Part model, mm, in its own coordinate system. A direction names the side the tool comes from. Coordinates: 2 decimals unless noted, no trailing zeros. Write each loop counter-clockwise with the first axis right and the second up, starting at its lowest first coordinate (ties: lowest second). Pieces come first, ordered by that corner, then holes. Notation, with made-up numbers: (35, 75) -> (66, 75) arc R26 cw to (66, 110) -> close; hole circle Ø10 at (-6.5, 19.5). An arc over 180 degrees is marked (long way). Write item = value, one per line.
from build123d import *

# Parameters (mm, degrees)
IZIM1_W                     = 40
IZIM1_H                     = 70
Y_KSEKLIK_EKSTR_ZYON1_DEPTH = 20
IZIM2_W                     = 18
IZIM2_H                     = 10
KES_EKSTR_ZYON1_DEPTH       = 71
IZIM3_W                     = 40
IZIM3_H                     = 20
Y_KSEKLIK_EKSTR_ZYON2_DEPTH = 5
IZIM4_W                     = 40
IZIM4_H                     = 20
Y_KSEKLIK_EKSTR_ZYON3_DEPTH = 20
IZIM5_W                     = 16
IZIM5_H                     = 10
KES_EKSTR_ZYON2_DEPTH       = 21


with BuildPart() as part:
    # Çizim1 → Yükseklik-Ekstrüzyon1 (new body)
    with BuildSketch(Plane(origin=(0, 0, 0), x_dir=(1, 0, 0), z_dir=(0, 1, 0))):
        Rectangle(IZIM1_W, IZIM1_H)
    extrude(amount=Y_KSEKLIK_EKSTR_ZYON1_DEPTH)

    # Çizim2 → Kes-Ekstrüzyon1 (cut, through all)
    with BuildSketch(Plane.XY.offset(35)):
        with Locations((0, 5)):
            Rectangle(IZIM2_W, IZIM2_H)
    extrude(amount=-KES_EKSTR_ZYON1_DEPTH, mode=Mode.SUBTRACT)

    # Çizim3 → Yükseklik-Ekstrüzyon2 (add)
    with BuildSketch(Plane(origin=(0, 20, 0), x_dir=(1, 0, 0), z_dir=(0, 1, 0))):
        with Locations((0, -25)):
            Rectangle(IZIM3_W, IZIM3_H)
    extrude(amount=Y_KSEKLIK_EKSTR_ZYON2_DEPTH)

    # Çizim4 → Yükseklik-Ekstrüzyon3 (add)
    with BuildSketch(Plane(origin=(0, 20, 0), x_dir=(1, 0, 0), z_dir=(0, 1, 0))):
        with Locations((0, 25)):
            Rectangle(IZIM4_W, IZIM4_H)
    extrude(amount=Y_KSEKLIK_EKSTR_ZYON3_DEPTH)

    # Çizim5 → Kes-Ekstrüzyon2 (cut, through all)
    with BuildSketch(Plane.XY.offset(-15)):
        with Locations((0, 35)):
            Rectangle(IZIM5_W, IZIM5_H)
    extrude(amount=-KES_EKSTR_ZYON2_DEPTH, mode=Mode.SUBTRACT)


solid = part.part
Q1. Mould opens along Z. For faces 1 (the face through (0, 22, 15)), 2 (the face through (8, 35, -25)), 3 (the face through (0, 20, 0)), 4 (the face through (0, 15, 35)) say: released by +Z, released by -Z, zero draft, split by the parting line, or undercut.
Model answer:
face_1 = undercut
face_2 = zero draft
face_3 = undercut
face_4 = released by +Z
Q2. Which spindle directions (+Z, -Z, +X, -X, +Y, -Y) get a long thin tool onto all of the face, cutting with end or side? Do faces 5 (the face through (0, 25, 25)), 6 (the face through (-8, 35, -25)), 7 (the face through (0, 28, -15)), 8 (the face through (9, 5, 0)). Say none if no direction does.
Model answer:
face_5 = +Z, +X, -X, +Y
face_6 = +Z, -Z, +Y
face_7 = +X, -X, +Y
face_8 = +Z, -Z, -Y
Q3. Saw through at D-D on y = 34. Give the cut face in (x, z).
Model answer:
outline = (-20, -35) -> (-8, -35) -> (-8, -15) -> (-20, -15) -> close; (8, -35) -> (20, -35) -> (20, -15) -> (8, -15) -> close
Q4. Pin check, flat tips, straight feed: pin 1 (16 mm diameter, centred on x = 3.5, y = 28.5, fed in from +Z); pin 2 (5 mm diameter, centred on x = 1, z = -21.5, fed in from +Y); pin 3 (16 mm diameter, centred on x = -0.5, z = 22.5, fed in from +Y). Stop position of each tip, or through.
Model answer:
pin_1 = 35
pin_2 = 30
pin_3 = 25
Q5. Saw through at C-C on z = 30. Give the cut face in (x, y).
Model answer:
outline = (-20, 0) -> (-9, 0) -> (-9, 10) -> (9, 10) -> (9, 0) -> (20, 0) -> (20, 25) -> (-20, 25) -> close
Q6. Saw through at B-B on x = 15.5. Give the cut face in (y, z), and give its area (3 significant figures).
Model answer:
outline = (0, -35) -> (40, -35) -> (40, -15) -> (20, -15) -> (20, 15) -> (25, 15) -> (25, 35) -> (0, 35) -> close
area = 1,900 mm²
Q7. Saw through at A-A on y = 23. Give the cut face in (x, z).
Model answer:
outline = (-20, -35) -> (20, -35) -> (20, -15) -> (-20, -15) -> close; (-20, 15) -> (20, 15) -> (20, 35) -> (-20, 35) -> close
Q8. Probe line 1 (X direction, y = 5, z = 12); line 2 (Z direction, x = 2, y = 22); line 3 (Y direction, x = 8.5, z = -25.5). List the from-to ranges inside material, lowest first. Write a range as from..to.
Model answer:
line_1 = -20..-9, 9..20
line_2 = -35..-15, 15..35
line_3 = 10..40
